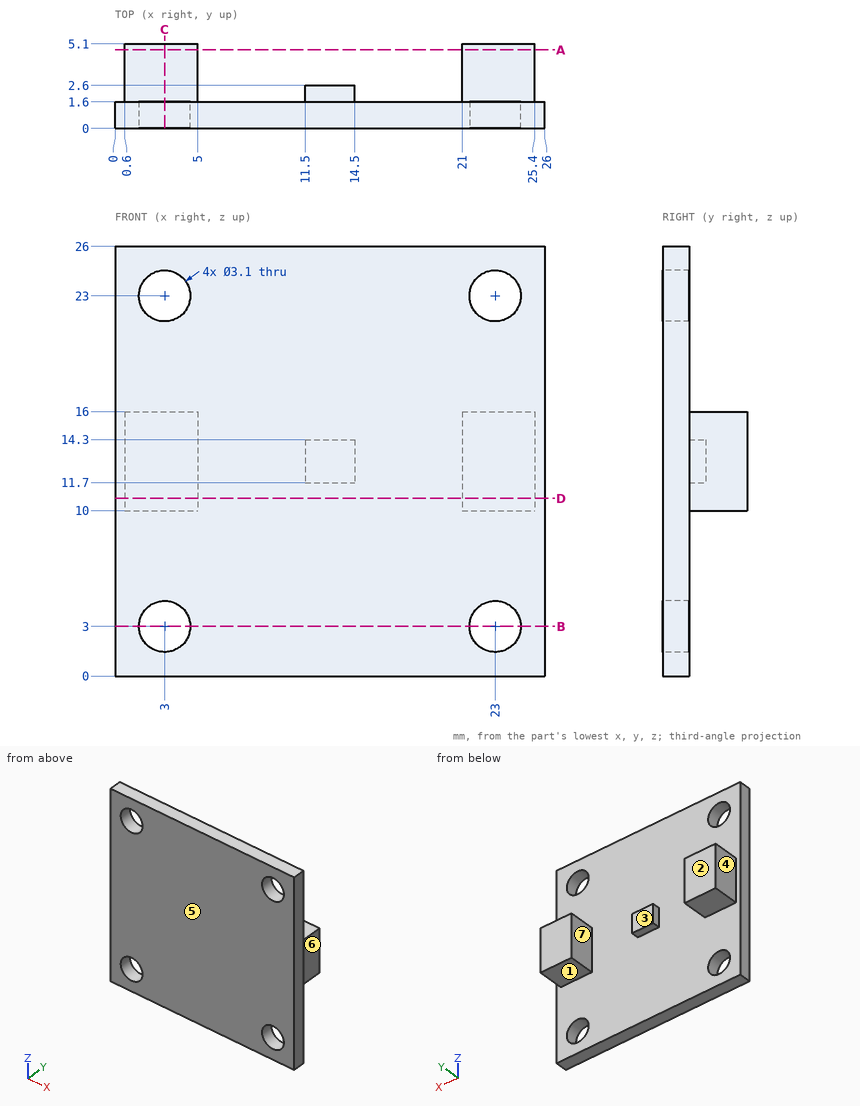
Part print with two shaded views. Sizes in mm from the minimum x, y, z corner. A direction names the side the tool comes from. Coordinates: 2 decimals unless noted, no trailing zeros. Write each loop counter-clockwise with the first axis right and the second up, starting at its lowest first coordinate (ties: lowest second). Pieces come first, ordered by that corner, then holes.
1. 3-axis set-ups, long thin cutter, end or side, ignore diameter. For the marked faces 1, 2, 3 and 4: which of +Z, -Z, +X, -X, +Y, -Y reach the whole face in a straight line?
Answer block:
face 1: -Z, +X, -X, +Y
face 2: +Z, -Z, +X, -X, +Y
face 3: +Z, -Z, +Y
face 4: +Z, -Z, -X, +Y
2. Drill centre lines: probe 1 along X at (y, z) = (0.8, 3); probe 2 along X at (y, z) = (1.55, 21.75). Where is each one in solid material? Low to high.
Answer block:
probe 1: x = 0 to 1.45, 4.55 to 21.45, 24.55 to 26
probe 2: x = 0 to 2.08, 3.92 to 22.08, 23.92 to 26
3. Band-saw the part on B-B, the plane z = 3. Give the cut face in (x, y).
Answer block:
outline: (0, 0) - (1.45, 0) - (1.45, 1.6) - (0, 1.6) - close; (4.55, 0) - (21.45, 0) - (21.45, 1.6) - (4.55, 1.6) - close; (24.55, 0) - (26, 0) - (26, 1.6) - (24.55, 1.6) - close
4. Band-saw the part on D-D, the plane z = 10.75. Give the cut face in (x, y).
Answer block:
outline: (0, 0) - (26, 0) - (26, 1.6) - (25.4, 1.6) - (25.4, 5.1) - (21, 5.1) - (21, 1.6) - (5, 1.6) - (5, 5.1) - (0.6, 5.1) - (0.6, 1.6) - (0, 1.6) - close
5. Pull direction X, two halves, no side cores. Call the marked faces 5, 6 and 7: released by +X, released by -X, zero draft, split by the parting line, or undercut.
Answer block:
face 5: zero draft
face 6: released by +X
face 7: undercut
6. Band-saw the part on A-A, the plane y = 4.75. Give the cut face in (x, z), and give its area (3 significant figures).
Answer block:
outline: (0.6, 10) - (5, 10) - (5, 16) - (0.6, 16) - close; (21, 10) - (25.4, 10) - (25.4, 16) - (21, 16) - close
area: 52.8 mm2
7. Band-saw the part on C-C, the plane x = 3. Give the cut face in (y, z).
Answer block:
outline: (0, 0) - (1.6, 0) - (1.6, 1.45) - (0, 1.45) - close; (0, 4.55) - (1.6, 4.55) - (1.6, 10) - (5.1, 10) - (5.1, 16) - (1.6, 16) - (1.6, 21.45) - (0, 21.45) - close; (0, 24.55) - (1.6, 24.55) - (1.6, 26) - (0, 26) - close
8. Drop flat-ended pins along their axis: pin 1 (4 mm diameter, centred on x = 3, z = 23, fed in from +Y); pin 2 (3 mm diameter, centred on x = 13.5, z = 17.5, fed in from -Y); pin 3 (1.3 mm diameter, centred on x = 13, z = 12.5, fed in from +Y); pin 4 (1.7 mm diameter, centred on x = 24, y = 3, fed in from +Z). Give the stop position or say it passes through.
Answer block:
pin 1: stops at y = 1.6
pin 2: stops at y = 0
pin 3: stops at y = 2.6
pin 4: stops at z = 16
